from build123d import *

# Parameters (mm, degrees)
SKETCH2_W               = 254
SKETCH2_H               = 101.6
BOSS_EXTRUDE1_DEPTH     = 4.7625
FILLET1_R               = 6.35
F_1_4_CLEARANCE_HOLE1_D = 6.7564
F_8_CLEARANCE_HOLE1_D   = 4.4958
F_4_CLEARANCE_HOLE1_D   = 3.2639


with BuildPart() as part:
    # Sketch2 → Boss-Extrude1 (new body)
    with BuildSketch(Plane(origin=(0, 0, 0), x_dir=(1, 0, 0), z_dir=(0, 1, 0))):
        with Locations((127, -50.8)):
            Rectangle(SKETCH2_W, SKETCH2_H)
    extrude(amount=BOSS_EXTRUDE1_DEPTH)

    # Fillet1
    fillet1_edges = [part.edges().sort_by_distance(p)[0] for p in [
        (0, 2.38125, 0),
        (254, 2.38125, 0),
        (254, 2.38125, 101.6),
        (0, 2.38125, 101.6),
    ]]
    fillet(fillet1_edges, radius=FILLET1_R)

    # 1/4 Clearance Hole1 (through all)
    with Locations(Plane(origin=(0, 4.7625, 0), x_dir=(1, 0, 0), z_dir=(0, 1, 0))):
        with Locations((12.7, -12.7), (12.7, -88.9), (241.3, -88.9), (241.3, -12.7)):
            Hole(F_1_4_CLEARANCE_HOLE1_D / 2)

    # #8 Clearance Hole1 (through all)
    with Locations(Plane(origin=(0, 4.7625, 0), x_dir=(1, 0, 0), z_dir=(0, 1, 0))):
        with Locations((142.24, -12.7), (215.9, -12.7), (215.9, -86.36), (142.24, -86.36)):
            Hole(F_8_CLEARANCE_HOLE1_D / 2)

    # #4 Clearance Hole1 (through all)
    with Locations(Plane(origin=(0, 4.7625, 0), x_dir=(1, 0, 0), z_dir=(0, 1, 0))):
        with Locations((38.1, -10.16), (102.87, -10.16), (102.87, -92.71), (38.1, -92.71)):
            Hole(F_4_CLEARANCE_HOLE1_D / 2)


solid = part.part
Geometry: final body of the model. Coordinates: model frame, mm. Round coordinates to 2 decimals unless told otherwise and drop trailing zeros. Order: outer loops, then holes, each group sorted by start corner. A loop starts at its lowest first (then second) coordinate and runs counter-clockwise, first axis right, second up. Notation, with made-up numbers: (41, -14.5) - (68, -14.5) arc R12 ccw to (68, 8.5) - close; hole circle Ø3 at (51.5, 88.25). An arc over 180 degrees is marked (long way). Write each question's results on one line, items separated by ' | '.
Item 1: Material intervals for line 1 along Z through (x, y) = (102.87, 2.45); line 2 along X through (y, z) = (1.9, 12.7); line 3 along X through (y, z) = (1, 92.71), sorted ascending. Write a range as [from, to].
Completed:
line 1: [0, 8.53], [11.79, 91.08], [94.34, 101.6] | line 2: [0, 9.32], [16.08, 139.99], [144.49, 213.65], [218.15, 237.92], [244.68, 254] | line 3: [0, 36.47], [39.73, 101.24], [104.5, 254]
Item 2: Section A-A, the plane x = 215.9. Return the cut outline in (y, z), and give its area (3 significant figures).
Completed:
outline: (0, 0) - (4.76, 0) - (4.76, 10.45) - (0, 10.45) - close; (0, 14.95) - (4.76, 14.95) - (4.76, 84.11) - (0, 84.11) - close; (0, 88.61) - (4.76, 88.61) - (4.76, 101.6) - (0, 101.6) - close | area: 441 mm^2
Item 3: First-contact query: pin 1 Ø1.5 at (x, z) = (84, 66) entering from -Y. Flat tip, straight axial feed; report the tip coordinate or a pass-through.
Completed:
pin 1: y = 0
Item 4: Mould query, pull axis Z, two halves, no side actions, for faces 1 (the cylindrical face through (213.824, 2.348, 87.221)), 2 (the flat face through (125, 2, 101.6)), 3 (the cylindrical face through (252.19, 2.41, 1.91)). Classes: pulls with the +Z half, pulls with the -Z half, needs draft (parallel to the pull), parting line crosses it, or undercut.
Completed:
face 1: undercut | face 2: pulls with the +Z half | face 3: pulls with the -Z half
